Model file for the job. Use its own axes, mm. A direction names the side the tool comes from. Round coordinates to 2 decimals unless told otherwise and drop trailing zeros. Order: outer loops, then holes, each group sorted by start corner. A loop starts at its lowest first (then second) coordinate and runs counter-clockwise, first axis right, second up. Notation, with made-up numbers: (14.5, 21) - (47.5, 21) arc R34 cw to (47.5, 58) - close; hole circle Ø9 at (21.25, 66.5). An arc over 180 degrees is marked (long way). Answer as CSV lines item,"result". Start each with the question number.
1. 3-axis set-ups, long thin cutter, end or side, ignore diameter. For faces 4 (the face through (85, 5, 8.75)), 5 (the face through (-79.5, 5, 0)), 6 (the face through (80.203, 9.285, -8.098)), 7 (the face through (80.152, 0.715, -8.047)): which of +Z, -Z, +X, -X, +Y, -Y reach the whole face in a straight line?
2. Band-saw the part on A-A on x = 62.5. List the corners of the cut face in (y, z).
3. Pull direction Z, two halves, no side cores. Call faces 1 (the face through (1, 4, 15)), 2 (the face through (88, 5, -11)), 3 (the face through (-85, 5, -8.75)): released by +Z, released by -Z, zero draft, split by the parting line, or undercut.
4. Band-saw the part on B-B on z = 0. List the corners of the cut face in (x, y), then the cut area to 3 significant figures.
5. Band-saw the part on C-C on y = 3.5. List the corners of the cut face in (x, z).
6. Wall check: line 1 along X through (y, z) = (4.15, 0); line 2 along X through (y, z) = (8.5, 5.25); line 3 along X through (y, z) = (1.75, -3.25). Give the ranges that are in metal, low to high. Write a range as [from, to].
7. Pin check, flat tips, straight feed: pin 1 Ø4.5 at (y, z) = (9, 5.5) entering from +X; pin 2 Ø12 at (x, z) = (11.5, 7) entering from +Y; pin 3 Ø5 at (x, z) = (-18, 2) entering from -Y; pin 4 Ø1.8 at (x, z) = (62, -11.5) entering from +Y. Stop position of each tip, or through.
8. Band-saw the part on D-D on x = -32. List the corners of the cut face in (y, z), then the cut area to 3 significant figures.
Autodesk Inventor part; units mm, degrees
ref_plane "YZ Plane" through (0, 0, 0) normal (1, 0, 0) x (0, 1, 0)
ref_plane "XZ Plane" through (0, 0, 0) normal (0, 1, 0) x (-1, 0, 0)
ref_plane "XY Plane" through (0, 0, 0) normal (0, 0, 1) x (1, 0, 0)
sketch "Body Outline" plane through (0, 0, 0) normal (0, 1, 0) x (-1, 0, 0)
  line L0 (88, -15) -> (-88, -15)
  line L1 (-88, -15) -> (-88, 15)
  line L2 (-88, 15) -> (88, 15)
  line L3 (88, 15) -> (88, -15)
  point P0 (0, 0)
  dimension "d0" = 30
  dimension "d1" = 15
  dimension "d2" = 176
  dimension "d3" = 88
extrude "Body" add sketch "Body Outline" along normal blind 10
sketch "Body Cutout Outline" plane through (0, 10, 0) normal (0, 1, 0) x (1, 0, 0)
  line L0 (-74, 15) -> (74, 15)
  line L1 (74, 15) -> (74, -15)
  line L2 (74, -15) -> (-74, -15)
  line L3 (-74, -15) -> (-74, 15)
  line L4 (-88, 15) -> (-88, -15)
  line L5 (88, -15) -> (88, 15)
  line L6 (88, 15) -> (-88, 15)
  line L7 (-88, -15) -> (88, -15)
  point P0 (0, 0)
  dimension "d6" = 14
  dimension "d7" = 14
  dimension "d8" = 0
  dimension "d9" = 0
extrude "Body Cutout" cut sketch "Body Cutout Outline" against normal blind 4 contours L0 L1 L2 L3
sketch "Rail Cutouts Outline" plane through (0, 0, 0) normal (0, -1, 0) x (1, 0, 0)
  line L0 (99.5, -8.75) -> (79.5, -8.75)
  line L1 (79.5, -8.75) -> (79.5, 8.75)
  line L2 (79.5, 8.75) -> (99.5, 8.75)
  line L3 (99.5, 8.75) -> (99.5, -8.75)
  line L4 (88, -15) -> (88, 15)
  line L5 (-99.5, -8.75) -> (-79.5, -8.75)
  line L6 (-79.5, -8.75) -> (-79.5, 8.75)
  line L7 (-79.5, 8.75) -> (-99.5, 8.75)
  line L8 (-99.5, 8.75) -> (-99.5, -8.75)
  line L9 (-88, 15) -> (-88, -15)
  point P0 (0, 0)
  dimension "d12" = 8.5
  dimension "d13" = 17.5
  dimension "d14" = 8.75
  dimension "d16" = 8.5
  dimension "d17" = 20
  dimension "d18" = 20
  dimension "d19" = 17.5
  dimension "d20" = 8.75
extrude "Rail Cutouts" cut sketch "Rail Cutouts Outline" along normal through all both and the other way through all
sketch "Spigot Cutouts Outline" plane through (0, 6, 0) normal (0, 1, 0) x (1, 0, 0)
  arc A0 (-65.5, 4.3084) -> (-59.5, 4.3084) centre (-62.5, 0) ccw
  line L0 (-65.5, 15) -> (-59.5, 15)
  line L1 (-59.5, 15) -> (-59.5, 4.3084)
  line L2 (-65.5, 4.3084) -> (-65.5, 15)
  line L3 (-74, 15) -> (74, 15)
  arc A1 (59.5, 4.3084) -> (65.5, 4.3084) centre (62.5, 0) ccw
  line L4 (59.5, 15) -> (65.5, 15)
  line L5 (65.5, 15) -> (65.5, 4.3084)
  line L6 (59.5, 4.3084) -> (59.5, 15)
  point P0 (0, 0)
  dimension "d23" = 6
  dimension "d24" = 62.5
  dimension "d25" = 0
  dimension "d26" = 0
  dimension "d27" = 5.25
  dimension "d28" = 3
  dimension "d29" = 6
  dimension "d30" = 3
  dimension "d31" = 5.25
  dimension "d32" = 0
  dimension "d33" = 0
  dimension "d34" = 62.5
extrude "Spigot Cutouts" cut sketch "Spigot Cutouts Outline" along normal through all both and the other way through all
sketch "Spigot Supports Outline" plane through (0, 0, 0) normal (0, -1, 0) x (1, 0, 0)
  line L0 (-65.5, -4.3084) -> (-59.5, -4.3084)
  line L1 (-59.5, -4.3084) -> (-59.5, -15)
  line L2 (-59.5, -15) -> (-65.5, -15)
  line L3 (-65.5, -15) -> (-65.5, -4.3084)
  line L4 (-65.5, -15) -> (-65.5, -4.3084)
  line L5 (-59.5, -4.3084) -> (-59.5, -15)
  line L6 (-88, -15) -> (-65.5, -15)
  line L7 (59.5, -4.3084) -> (65.5, -4.3084)
  line L8 (65.5, -4.3084) -> (65.5, -15)
  line L9 (65.5, -15) -> (59.5, -15)
  line L10 (59.5, -15) -> (59.5, -4.3084)
  line L11 (65.5, -4.3084) -> (65.5, -15)
  line L12 (59.5, -15) -> (59.5, -4.3084)
  line L13 (-59.5, -15) -> (59.5, -15)
  point P0 (0, 0)
  dimension "d37" = 0
  dimension "d38" = 0
  dimension "d39" = 0
  dimension "d40" = 0
  dimension "d41" = 0
  dimension "d42" = 0
  dimension "d43" = 0
  dimension "d44" = 0
extrude "Spigot Supports" add sketch "Spigot Supports Outline" against normal blind 2
fillet "Body Fillet" radius 3 4 edges at (-79.5, 5, -8.75) (-79.5, 5, 8.75) (79.5, 5, -8.75) (79.5, 5, 8.75)
fillet "Body Fillet" radius 2 4 edges at (-88, 5, 15) (-88, 5, -15) (88, 5, -15) (88, 5, 15)
chamfer "Rail Cutouts Chamfer" distance 1 angle 45 20 edges at (-85.25, 10, -8.75) (-80.3787, 10, -7.8713) (-79.5, 10, 0) (-80.3787, 10, 7.8713) (-85.25, 10, 8.75) (-85.25, 0, -8.75) (-80.3787, 0, -7.8713) (-79.5, 0, 0) (-80.3787, 0, 7.8713) (-85.25, 0, 8.75) (85.25, 10, -8.75) (80.3787, 10, -7.8713) (79.5, 10, 0) (80.3787, 10, 7.8713) (85.25, 10, 8.75) (85.25, 0, 8.75) (80.3787, 0, 7.8713) (79.5, 0, 0) (80.3787, 0, -7.8713) (85.25, 0, -8.75)
equation "\"d7\" = d6"
equation "\"d16\" = d12"
equation "\"d18\" = d17"
equation "\"d19\" = d13"
equation "\"d28\" = 0.5 * d23"
equation "\"d29\" = d23"
equation "\"d30\" = d28"
equation "\"d31\" = d27"
properties part number "LR Spigot Plate" material "Acetal Resin, Black"
Reply:
1,face 4,"+X, +Y, -Y"
1,face 5,"-X, +Y, -Y"
1,face 6,"+X, +Y"
1,face 7,"+X, -Y"
2,outline,"(0, -15) - (2, -15) - (2, -4.31) - (0, -4.31) - close; (0, 5.25) - (6, 5.25) - (6, 15) - (0, 15) - close"
3,face 1,"released by +Z"
3,face 2,"zero draft"
3,face 3,"undercut"
4,outline,"(-79.5, 1) - (-78.5, 0) - (-67.75, 0) - (-67.75, 6) - (-74, 6) - (-74, 10) - (-78.5, 10) - (-79.5, 9) - close; (-57.25, 0) - (57.25, 0) - (57.25, 6) - (-57.25, 6) - close; (67.75, 0) - (78.5, 0) - (79.5, 1) - (79.5, 9) - (78.5, 10) - (74, 10) - (74, 6) - (67.75, 6) - close"
4,area,"870 mm2"
5,outline,"(-88, -13) arc R2 ccw to (-86, -15) - (-65.5, -15) - (-65.5, -4.31) arc R5.25 cw (long way) to (-59.5, -4.31) - (-59.5, -15) - (59.5, -15) - (59.5, -4.31) arc R5.25 cw (long way) to (65.5, -4.31) - (65.5, -15) - (86, -15) arc R2 ccw to (88, -13) - (88, -8.75) - (82.5, -8.75) arc R3 cw to (79.5, -5.75) - (79.5, 5.75) arc R3 cw to (82.5, 8.75) - (88, 8.75) - (88, 13) arc R2 ccw to (86, 15) - (-86, 15) arc R2 ccw to (-88, 13) - (-88, 8.75) - (-82.5, 8.75) arc R3 cw to (-79.5, 5.75) - (-79.5, -5.75) arc R3 cw to (-82.5, -8.75) - (-88, -8.75) - close"
6,line 1,"x = [-79.5, -67.75], [-57.25, 57.25], [67.75, 79.5]"
6,line 2,"x = [-79.5, -74], [74, 79.5]"
6,line 3,"x = [-79.5, -66.62], [-58.38, 58.38], [66.62, 79.5]"
7,pin 1,"stops at x = 80.26"
7,pin 2,"stops at y = 6"
7,pin 3,"stops at y = 0"
7,pin 4,"stops at y = 2"
8,outline,"(0, -15) - (6, -15) - (6, 15) - (0, 15) - close"
8,area,"180 mm2"
